Autodesk Inventor part; units mm, degrees
ref_plane "YZ Plane" through (0, 0, 0) normal (1, 0, 0) x (0, 1, 0)
ref_plane "XZ Plane" through (0, 0, 0) normal (0, 1, 0) x (-1, 0, 0)
ref_plane "XY Plane" through (0, 0, 0) normal (0, 0, 1) x (1, 0, 0)
sketch "Sketch7" plane through (0, 0, 0) normal (0, 1, 0) x (-1, 0, 0)
  line L0 (-25, -25) -> (25, -25)
  line L1 (25, -25) -> (25, 25)
  line L2 (25, 25) -> (-25, 25)
  line L3 (-25, 25) -> (-25, -25)
  line L4 (-25, -25) -> (25, 25) construction
  line L5 (25, -25) -> (-25, 25) construction
  point P0 (0, 0)
  point P1 (0, 0)
  dimension "d54" = 50
  dimension "d55" = 50
extrude "Extrusion4" add sketch "Sketch7" along normal blind 3
sketch "Sketch8" plane through (0, 3, 0) normal (0, 1, 0) x (1, 0, 0)
  circle A0 centre (0, 0) radius 21
  dimension "d58" = 42
extrude "Extrusion5" cut sketch "Sketch8" against normal blind 3
sketch "Sketch10" plane through (0, 3, 0) normal (0, 1, 0) x (1, 0, 0)
  line L0 (-18, -18) -> (18, -18)
  line L1 (18, -18) -> (18, 18)
  line L2 (18, 18) -> (-18, 18)
  line L3 (-18, 18) -> (-18, -18)
  line L4 (-18, -18) -> (18, 18) construction
  line L5 (18, -18) -> (-18, 18) construction
  point P0 (0, 0)
  dimension "d62" = 36
  dimension "d63" = 36
hole "Hole2" at (-18, 3, 18) at (-18, 3, -18) at (18, 3, -18) at (18, 3, 18) direction (0, -1, 0) diameter 3.264 end through all
properties part number "chamberPlateNA11_thin"
Input: part model. Units: mm. Frame: model coordinates. Give positions to 0.01 mm unless a question says otherwise; leave off trailing zeros. Order: outer loops, then holes, each group sorted by start corner. A loop starts at its lowest first (then second) coordinate and runs counter-clockwise, first axis right, second up.
1. Pin query (flat end, axial travel): pin 1 (2 mm diameter, centred on x = -18, z = 18, fed in from +Y). Return the tip coordinate at first contact, or that it passes through.
Derived:
pin 1: passes through
2. Section C-C on z = 17. Return the cut outline in (x, y).
Derived:
outline: (-25, 0) - (-19.29, 0) - (-19.29, 3) - (-25, 3) - close; (-16.71, 0) - (-12.33, 0) - (-12.33, 3) - (-16.71, 3) - close; (12.33, 0) - (16.71, 0) - (16.71, 3) - (12.33, 3) - close; (19.29, 0) - (25, 0) - (25, 3) - (19.29, 3) - close
3. Material intervals for L1, parallel to Z at x = 17, y = 1.9; L2, parallel to Z at x = 0, y = 1.3; L3, parallel to X at y = 1.9, z = 18, sorted ascending.
Derived:
L1: z = -25 to -19.29, -16.71 to -12.33, 12.33 to 16.71, 19.29 to 25
L2: z = -25 to -21, 21 to 25
L3: x = -25 to -19.63, -16.37 to -10.82, 10.82 to 16.37, 19.63 to 25
4. Section A-A on x = 0. Return the cut outline in (y, z), and give its area (3 significant figures).
Derived:
outline: (0, -25) - (3, -25) - (3, -21) - (0, -21) - close; (0, 21) - (3, 21) - (3, 25) - (0, 25) - close
area: 24.0 mm2
5. Section B-B on y = 0.65. Return the cut outline in (x, z).
Derived:
outline: (-25, -25) - (25, -25) - (25, 25) - (-25, 25) - close; hole circle Ø42 at (0, 0); hole circle Ø3.26 at (-18, -18); hole circle Ø3.26 at (-18, 18); hole circle Ø3.26 at (18, -18); hole circle Ø3.26 at (18, 18)
6. Mould query, pull axis X, two halves, no side actions, for faces 1 (the flat face through (-25, 1, 0)), 2 (the flat face through (0, 1, 25)), 3 (the cylindrical face through (17.93, 1.48, 16.37)). Classes: released by +X, released by -X, zero draft, split by the parting line, or undercut.
Derived:
face 1: released by -X
face 2: zero draft
face 3: undercut
7. Section D-D on x = -18. Return the cut outline in (y, z), and give its area (3 significant figures).
Derived:
outline: (0, -25) - (3, -25) - (3, -19.63) - (0, -19.63) - close; (0, -16.37) - (3, -16.37) - (3, -10.82) - (0, -10.82) - close; (0, 10.82) - (3, 10.82) - (3, 16.37) - (0, 16.37) - close; (0, 19.63) - (3, 19.63) - (3, 25) - (0, 25) - close
area: 65.5 mm2
